Geometry: final body of the model. Coordinates: model frame, mm. A direction names the side the tool comes from. Coordinates: 2 decimals unless noted, no trailing zeros. Order: outer loops, then holes, each group sorted by start corner. A loop starts at its lowest first (then second) coordinate and runs counter-clockwise, first axis right, second up. Notation, with made-up numbers: M 14.5,5.5 L 68.5,5.5 A34 ccw 68.5,44.5 Z; hole C -30.75,55 d9. An arc over 180 degrees is marked long. Write item = value, one per line.
from build123d import *

# Parameters (mm, degrees)
CUT_EXTRUDE1_START = 4
CUT_EXTRUDE1_DEPTH = 10


with BuildPart() as part:
    # Sketch1 → Revolve1 (revolve)
    with BuildSketch(Plane.XY):
        Polygon((0, 0), (0, 3.5), (10, 3.5), (10, 4), (17, 4), (17, 4.5), (29, 4.5), (29, 0), align=None)
    revolve(axis=Axis((29, 0, 0), (-1, 0, 0)))

    # Sketch2 → Cut-Extrude1 (cut)
    with BuildSketch(Plane(origin=(0, 0, 0), x_dir=(1, 0, 0), z_dir=(0, 1, 0)).offset(CUT_EXTRUDE1_START)):
        with BuildLine():
            Line((19.76662124, 1.5), (26.76662124, 1.5))
            ThreePointArc((26.76662124, 1.5), (28.26662124, 0), (26.76662124, -1.5))
            Line((26.76662124, -1.5), (19.76662124, -1.5))
            ThreePointArc((19.76662124, -1.5), (18.26662124, 0), (19.76662124, 1.5))
        make_face()
    extrude(amount=CUT_EXTRUDE1_DEPTH, mode=Mode.SUBTRACT)


solid = part.part
1) Mould query, pull axis Y, two halves, no side actions, for faces 1 (the face through (23, 4, 0)), 2 (the face through (13.549, -0.867, 3.905)), 3 (the face through (29, 0, 0)). Classes: pulls with the +Y half, pulls with the -Y half, needs draft (parallel to the pull), parting line crosses it, or undercut.
Numbers:
face_1 = pulls with the +Y half
face_2 = parting line crosses it
face_3 = needs draft
2) Section A-A, the plane y = 0. Return loops of the section in (x, z), and give its area (3 significant figures).
Numbers:
outline = M 0,-3.5 L 10,-3.5 L 10,-4 L 17,-4 L 17,-4.5 L 29,-4.5 L 29,4.5 L 17,4.5 L 17,4 L 10,4 L 10,3.5 L 0,3.5 Z
area = 234 mm²
3) Section D-D, the plane y = 2.5. Return loops of the section in (x, z), and give its area (3 significant figures).
Numbers:
outline = M 0,-2.45 L 10,-2.45 L 10,-3.12 L 17,-3.12 L 17,-3.74 L 29,-3.74 L 29,3.74 L 17,3.74 L 17,3.12 L 10,3.12 L 10,2.45 L 0,2.45 Z
area = 183 mm²
4) Pin query (flat end, axial travel): pin 1 (4 mm diameter, centred on x = 21.5, y = -3, fed in from -Z); pin 2 (1.5 mm diameter, centred on x = 14.5, y = 2.5, fed in from +Z); pin 3 (0.9 mm diameter, centred on x = 23, z = 0, fed in from +Y). Return the tip coordinate at first contact, or that it passes through.
Numbers:
pin_1 = -4.39
pin_2 = 3.6
pin_3 = 4
5) Section B-B, the plane z = 0. Return loops of the section in (x, y).
Numbers:
outline = M 0,-3.5 L 10,-3.5 L 10,-4 L 17,-4 L 17,-4.5 L 29,-4.5 L 29,4.5 L 28.27,4.5 L 28.27,4 L 18.27,4 L 18.27,4.5 L 17,4.5 L 17,4 L 10,4 L 10,3.5 L 0,3.5 Z
6) Section C-C, the plane x = 13.5. Return loops of the section in (y, z).
Numbers:
outline = C 0,0 d8
7) Set-up query: faces 4 (the face through (18.267, 4.191, 0.033)), 5 (the face through (0, 0, 0)), 6 (the face through (5.07, 3.233, 1.341)). Return all of +Z, -Z, +X, -X, +Y, -Y with unobstructed straight access to the full face (end or side cutting, diameter ignored); none if empty.
Numbers:
face_4 = +Y
face_5 = +Z, -Z, -X, +Y, -Y
face_6 = -X
8) Line query: L1, parallel to Y at x = 11.25, z = 0; L2, parallel to X at y = -3.25, z = 1.75; L3, parallel to X at y = 2.5, z = 3.25. Output: solid intervals per line, ascending.
Numbers:
L1 = -4 to 4
L2 = 10 to 29
L3 = 17 to 29
